from build123d import *

# Parameters (mm, degrees)
SKETCH_1_W      = 6.1
SKETCH_1_H      = 6.1
SKETCH_1_R      = 9.55
SKETCH_1_R_2    = 2.1
EXTRUDE_2_DEPTH = 2
FILLET_1_R      = 45
FILLET_2_R      = 10


with BuildPart() as part:
    # 草图1 → 凸台-拉伸2 (new body)
    with BuildSketch(Plane.XY):
        with BuildLine():
            Line((-10.195923298, 166.045688989), (-10.195923298, 93.338899377))
            Line((-10.195923298, 93.338899377), (-10.195923298, -3.112918115))
            Line((-10.195923298, -3.112918115), (6.754076702, -25.161100623))
            ThreePointArc((6.754076702, -25.161100623), (31.304076702, -49.711100623), (55.854076702, -25.161100623))
            Line((55.854076702, -25.161100623), (61.387071712, 1.202006387))
            Line((61.387071712, 1.202006387), (61.387071712, 34.710258927))
            Line((61.387071712, 34.710258927), (52.804076702, 50.954174352))
            Line((52.804076702, 50.954174352), (52.804076702, 93.338899377))
            Line((52.804076702, 93.338899377), (52.804076702, 205.407441872))
            Line((52.804076702, 205.407441872), (1.570402993, 233.385501559))
            ThreePointArc((1.570402993, 233.385501559), (-33.983226461, 217.910695504), (-10.195923298, 187.288899377))
            Line((-10.195923298, 187.288899377), (-10.195923298, 166.045688989))
        make_face()
        with Locations((10.304076702, 14.560258927)):
            Rectangle(SKETCH_1_W, SKETCH_1_H, mode=Mode.SUBTRACT)
        with Locations((10.304076702, 31.660258927)):
            Rectangle(SKETCH_1_W, SKETCH_1_H, mode=Mode.SUBTRACT)
        with Locations((31.304076702, -25.161100623)):
            Circle(SKETCH_1_R, mode=Mode.SUBTRACT)
        with Locations((26.304076702, 19.560258927)):
            Circle(SKETCH_1_R_2, mode=Mode.SUBTRACT)
        with Locations((36.304076702, 19.560258927)):
            Circle(SKETCH_1_R_2, mode=Mode.SUBTRACT)
        with Locations((52.304076702, 14.560258927)):
            Rectangle(SKETCH_1_W, SKETCH_1_H, mode=Mode.SUBTRACT)
        with Locations((52.304076702, 31.660258927)):
            Rectangle(SKETCH_1_W, SKETCH_1_H, mode=Mode.SUBTRACT)
        Polygon((7.355428358, 168.902414276), (3.042076993, 164.589062911), (-1.271274372, 168.902414276), (3.042076993, 173.215765641), align=None, mode=Mode.SUBTRACT)
        with Locations((-10.195923298, 211.838899377)):
            Circle(SKETCH_1_R, mode=Mode.SUBTRACT)
        Polygon((19.446954316, 156.810888318), (15.133602951, 152.497536952), (10.820251586, 156.810888318), (15.133602951, 161.124239683), align=None, mode=Mode.SUBTRACT)
        with Locations((17.891319398, 176.680588869)):
            Circle(SKETCH_1_R_2, mode=Mode.SUBTRACT)
        with Locations((24.96238721, 183.751656681)):
            Circle(SKETCH_1_R_2, mode=Mode.SUBTRACT)
        Polygon((32.740561803, 202.914250451), (37.053913168, 198.600899086), (32.740561803, 194.28754772), (28.427210437, 198.600899086), align=None, mode=Mode.SUBTRACT)
        Polygon((49.145439126, 186.509373127), (44.832087761, 182.196021762), (40.518736396, 186.509373127), (44.832087761, 190.822724493), align=None, mode=Mode.SUBTRACT)
    extrude(amount=EXTRUDE_2_DEPTH)

    # 圆角1
    fillet_1_edges = [part.edges().sort_by_distance(p)[0] for p in [
        (-10.195923298, -3.112918115, 1),
        (52.804076702, 205.407441872, 1),
        (52.804076702, 50.954174352, 1),
        (6.754076702, -25.161100623, 1),
    ]]
    fillet(fillet_1_edges, radius=FILLET_1_R)

    # 圆角2
    fillet_2_edges = [part.edges().sort_by_distance(p)[0] for p in [
        (-10.195923298, 187.288899377, 1),
    ]]
    fillet(fillet_2_edges, radius=FILLET_2_R)


solid = part.part
The listing builds one solid part. Answer for the finished solid, in the listing's coordinates (mm). Coordinates: 2 decimals unless noted, no trailing zeros. Write each loop counter-clockwise with the first axis right and the second up, starting at its lowest first coordinate (ties: lowest second). Pieces come first, ordered by that corner, then holes. Notation, with made-up numbers: (64, 34) -> (94, 34) arc R23 cw to (94, 49) -> close; hole circle Ø8 at (7.25, -35). An arc over 180 degrees is marked (long way). One line per question, with ' | ' between items.
1. Section B-B (z = 0.6) is taken. State how many separate pieces and enclosed holes the cut face has, and give its area (3 significant figures).
Verdict:
separate pieces: 1 | enclosed holes: 14 | area: 16,800 mm^2
2. Given pin 1 Ø12 at (x, y) = (-2, 59) entering from -Z; pin 2 Ø0.6 at (y, z) = (33, 1) entering from -X; pin 3 Ø1 at (x, z) = (10.5, 1.5) entering from +Y, each flat-ended and moving along its own axis, determine where each tip first touches the part or whether it passes through.
Verdict:
pin 1: stops at z = 0 | pin 2: stops at x = -10.2 | pin 3: stops at y = 228.78
3. Section C-C (y = 65) is taken. Determine the outline of the cut face in (x, z), and give its area (3 significant figures).
Verdict:
outline: (-10.2, 0) -> (52.8, 0) -> (52.8, 2) -> (-10.2, 2) -> close | area: 126 mm^2
4. Section A-A (x = -4) is taken. Determine the outline of the cut face in (y, z).
Verdict:
outline: (-10.6, 0) -> (204.57, 0) -> (204.57, 2) -> (-10.6, 2) -> close; (219.11, 0) -> (235.59, 0) -> (235.59, 2) -> (219.11, 2) -> close
5. For a pull along Y with two mould halves and no side action, classify faces 1 (the cylindrical face through (40.126, -28.819, 0.986)), 2 (the cylindrical face through (46.33, 201.96, 1.01)), 3 (the flat face through (13, 95, 2)) as released by +Y, released by -Y, zero draft, split by the parting line, or undercut.
Verdict:
face 1: undercut | face 2: released by +Y | face 3: zero draft
6. Straight lines are drawn through the part: line 1 (X direction, y = 30, z = 1.35); line 2 (Y direction, x = 9, z = 0.15); line 3 (X direction, y = 69, z = 0.15). For each, find the intervals that lie inside material, in ascending order.
Verdict:
line 1: x = -10.2 to 7.25, 13.35 to 49.25, 55.35 to 61.39 | line 2: y = -35.42 to 11.51, 17.61 to 28.61, 34.71 to 229.33 | line 3: x = -10.2 to 52.8
7. Section D-D (x = -22.5) is taken. Determine the outline of the cut face in (y, z), and give its area (3 significant figures).
Verdict:
outline: (190.59, 0) -> (233.08, 0) -> (233.08, 2) -> (190.59, 2) -> close | area: 85.0 mm^2
